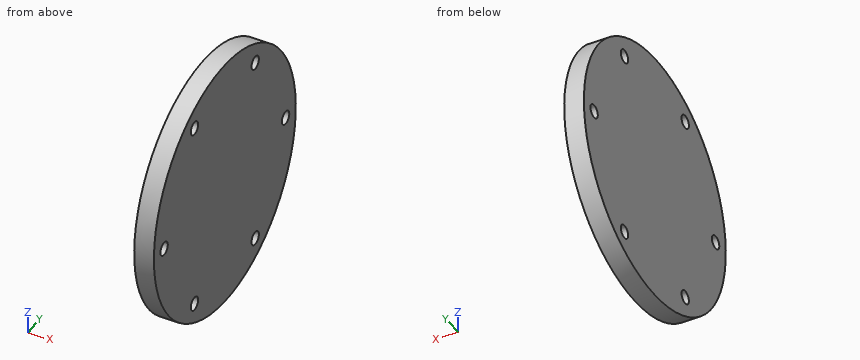
```python
from build123d import *

# Parameters (mm, degrees)
CROQUIS1_R                       = 32.7
SALIENTE_EXTRUIR1_DEPTH          = 5
TALADRO_DE_MARGEN_PARA_M31_D     = 3.4
TALADRO_DE_MARGEN_PARA_M31_DEPTH = 10
TALADRO_DE_MARGEN_PARA_M31_TIP   = 1.021463052


with BuildPart() as part:
    # Croquis1 → Saliente-Extruir1 (new body)
    with BuildSketch(Plane(origin=(0, 0, 0), x_dir=(0, 0, -1), z_dir=(1, 0, 0))):
        Circle(CROQUIS1_R)
    extrude(amount=SALIENTE_EXTRUIR1_DEPTH)

    # Taladro de margen para M31
    with Locations(Plane(origin=(5, 0, 0), x_dir=(0, 0, -1), z_dir=(1, 0, 0))):
        with Locations((0, 28), (24.248711306, 14), (24.248711306, -14), (0, -28), (-24.248711306, -14), (-24.248711306, 14)):
            Hole(TALADRO_DE_MARGEN_PARA_M31_D / 2, depth=TALADRO_DE_MARGEN_PARA_M31_DEPTH)
            with Locations((0, 0, -(TALADRO_DE_MARGEN_PARA_M31_DEPTH + TALADRO_DE_MARGEN_PARA_M31_TIP / 2))):  # 118° drill point
                Cone(0, TALADRO_DE_MARGEN_PARA_M31_D / 2, TALADRO_DE_MARGEN_PARA_M31_TIP, mode=Mode.SUBTRACT)


solid = part.part
```
Build history of the part. All positions in model axes, mm. Coordinates: 2 decimals unless noted, no trailing zeros. Order: outer loops, then holes, each group sorted by start corner. A loop starts at its lowest first (then second) coordinate and runs counter-clockwise, first axis right, second up.
Item 1: Drop flat-ended pins along their axis: pin 1 Ø3 at (x, y) = (0.5, -15.5) entering from +Z; pin 2 Ø3 at (x, z) = (2, 10) entering from -Y. Give the stop position or say it passes through.
Filled in:
pin 1: stops at z = 29.55
pin 2: stops at y = -31.58
Item 2: Saw through at A-A on z = 0. List the corners of the cut face in (x, y), then the cut area to 3 significant figures.
Filled in:
outline: (0, -32.7) - (5, -32.7) - (5, -29.7) - (0, -29.7) - close; (0, -26.3) - (5, -26.3) - (5, 26.3) - (0, 26.3) - close; (0, 29.7) - (5, 29.7) - (5, 32.7) - (0, 32.7) - close
area: 293 mm2
Item 3: Saw through at D-D on y = 28. List the corners of the cut face in (x, z).
Filled in:
outline: (0, -16.89) - (5, -16.89) - (5, -1.7) - (0, -1.7) - close; (0, 1.7) - (5, 1.7) - (5, 16.89) - (0, 16.89) - close
Item 4: Saw through at C-C on y = 14. List the corners of the cut face in (x, z), then the cut area to 3 significant figures.
Filled in:
outline: (0, -29.55) - (5, -29.55) - (5, -25.95) - (0, -25.95) - close; (0, -22.55) - (5, -22.55) - (5, 22.55) - (0, 22.55) - close; (0, 25.95) - (5, 25.95) - (5, 29.55) - (0, 29.55) - close
area: 262 mm2
Item 5: Drill centre lines: L1, parallel to Y at x = 2, z = 0; L2, parallel to Y at x = 4.05, z = 24.5; L3, parallel to Z at x = 4.6, y = 28.5. Where is each one in solid material? Low to high.
Filled in:
L1: y = -32.7 to -29.7, -26.3 to 26.3, 29.7 to 32.7
L2: y = -21.66 to -15.68, -12.32 to 12.32, 15.68 to 21.66
L3: z = -16.03 to -1.62, 1.62 to 16.03
Item 6: Saw through at B-B on x = 2.65. List the corners of the cut face in (y, z), then the cut area to 3 significant figures.
Filled in:
outline: circle Ø65.4 at (0, 0); hole circle Ø3.4 at (-28, 0); hole circle Ø3.4 at (-14, -24.25); hole circle Ø3.4 at (-14, 24.25); hole circle Ø3.4 at (14, -24.25); hole circle Ø3.4 at (14, 24.25); hole circle Ø3.4 at (28, 0)
area: 3,300 mm2
